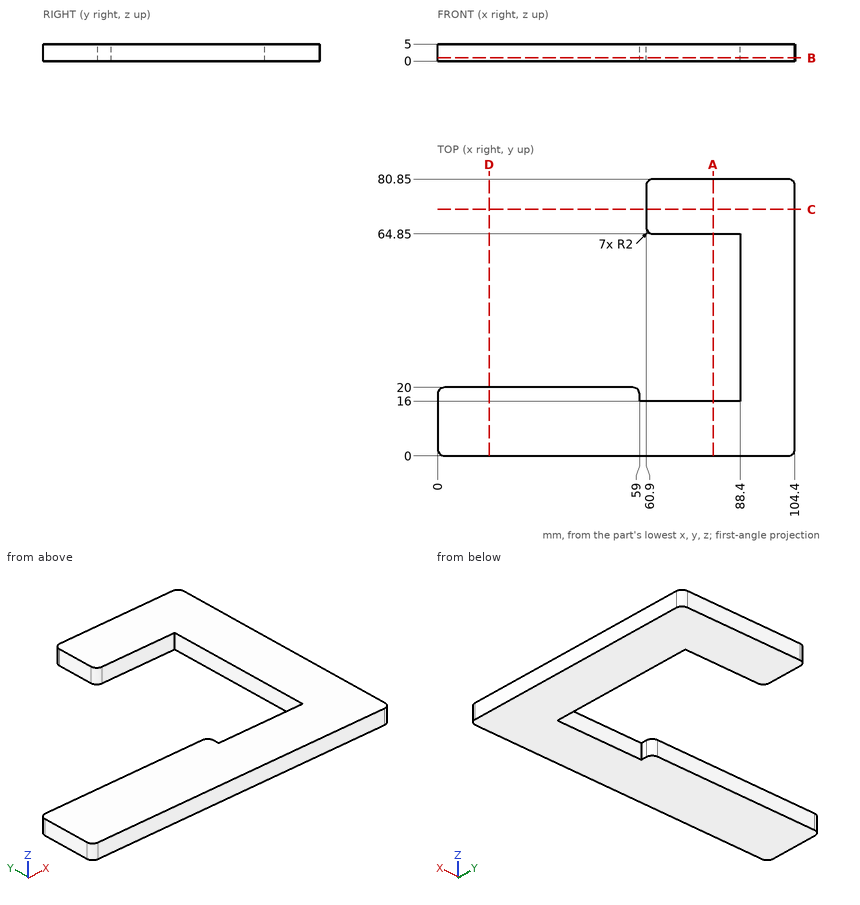
Source: three-view drawing plus pictorial views. Frame: mm from the lowest corner of the part. Round coordinates to 2 decimals unless told otherwise and drop trailing zeros. Write each loop counter-clockwise with the first axis right and the second up, starting at its lowest first coordinate (ties: lowest second). Pieces come first, ordered by that corner, then holes. Notation, with made-up numbers: (8, 42.25) -> (57, 42.25) arc R13 cw to (57, 55.25) -> close; hole circle Ø11 at (9, -18.75). An arc over 180 degrees is marked (long way). Return JSON: item names as keys, results as strings.
Q1. Section B-B on z = 0.95. Return the cut outline in (x, y).
From the geometry:
{"outline": "(0, 2) arc R2 ccw to (2, 0) -> (102.4, 0) arc R2 ccw to (104.4, 2) -> (104.4, 78.85) arc R2 ccw to (102.4, 80.85) -> (62.9, 80.85) arc R2 ccw to (60.9, 78.85) -> (60.9, 66.85) arc R2 ccw to (62.9, 64.85) -> (88.4, 64.85) -> (88.4, 16) -> (59, 16) -> (59, 18) arc R2 ccw to (57, 20) -> (2, 20) arc R2 ccw to (0, 18) -> close"}
Q2. Ray query, line 1 (Y direction, x = 81, z = 1.7); line 2 (Y direction, x = 56.5, z = 1.6); line 3 (X direction, y = 48, z = 4.6). Return the intervals inside material, ascending.
From the geometry:
{"line 1": "0 to 16, 64.85 to 80.85", "line 2": "0 to 20", "line 3": "88.4 to 104.4"}
Q3. First-contact query: pin 1 Ø12 at (x, y) = (65.5, 18.5) entering from +Z; pin 2 Ø1.5 at (x, z) = (32.5, 3.5) entering from +Y; pin 3 Ø3 at (y, z) = (60, 2) entering from -X. Flat tips, straight axial feed; report the tip coordinate or a pass-through.
From the geometry:
{"pin 1": "z = 5", "pin 2": "y = 20", "pin 3": "x = 88.4"}
Q4. Section D-D on x = 15. Return the cut outline in (y, z), and give its area (3 significant figures).
From the geometry:
{"outline": "(0, 0) -> (20, 0) -> (20, 5) -> (0, 5) -> close", "area": "100 mm2"}
Q5. Section A-A on x = 80.5. Return the cut outline in (y, z), and give its area (3 significant figures).
From the geometry:
{"outline": "(0, 0) -> (16, 0) -> (16, 5) -> (0, 5) -> close; (64.85, 0) -> (80.85, 0) -> (80.85, 5) -> (64.85, 5) -> close", "area": "160 mm2"}
Q6. Section C-C on y = 72. Return the cut outline in (x, z).
From the geometry:
{"outline": "(60.9, 0) -> (104.4, 0) -> (104.4, 5) -> (60.9, 5) -> close"}
